Geometry: final body of the model. Coordinates: model frame, mm. A direction names the side the tool comes from. Give positions to 0.01 mm unless a question says otherwise; leave off trailing zeros. Write each loop counter-clockwise with the first axis right and the second up, starting at its lowest first coordinate (ties: lowest second). Pieces come first, ordered by that corner, then holes. Notation, with made-up numbers: (11, 70) - (53, 70) arc R33 cw to (53, 106) - close; hole circle Ø3 at (-21.5, -19.75). An arc over 180 degrees is marked (long way). Return JSON: item names as keys, results as strings.
from build123d import *

# Parameters (mm, degrees)
SKETCH1_W                 = 96.9
SKETCH1_H                 = 214
BOSS_EXTRUDE1_DEPTH       = 3
SKETCH2_W                 = 7
SKETCH2_H                 = 214
CUT_EXTRUDE1_DEPTH        = 1.5
F_0_80_TAPPED_HOLE1_D     = 1.19126
F_0_80_TAPPED_HOLE1_DEPTH = 4.0005
F_0_80_TAPPED_HOLE1_TIP   = 0.357890611


with BuildPart() as part:
    # Sketch1 → Boss-Extrude1 (new body)
    with BuildSketch(Plane(origin=(0, 0, 0), x_dir=(1, 0, 0), z_dir=(0, 1, 0))):
        Rectangle(SKETCH1_W, SKETCH1_H)
    extrude(amount=BOSS_EXTRUDE1_DEPTH)

    # Sketch2 → Cut-Extrude1 (cut)
    with BuildSketch(Plane(origin=(0, 3, 0), x_dir=(1, 0, 0), z_dir=(0, 1, 0))):
        with Locations((44.95, 0)):
            Rectangle(SKETCH2_W, SKETCH2_H)
        with Locations((-44.95, 0)):
            Rectangle(SKETCH2_W, SKETCH2_H)
    extrude(amount=-CUT_EXTRUDE1_DEPTH, mode=Mode.SUBTRACT)

    # #0-80 Tapped Hole1
    with Locations(Plane(origin=(0, 3, 0), x_dir=(1, 0, 0), z_dir=(0, 1, 0))):
        with Locations((45.7, -102), (-45.8, -102), (45.7, -79.333333333), (-45.8, -79.333333333), (45.7, -56.666666667), (-45.8, -56.666666667), (45.7, -34), (-45.8, -34), (45.7, -11.333333333), (-45.8, -11.333333333), (45.7, 11.333333333), (-45.8, 11.333333333), (45.7, 34), (-45.8, 34), (45.7, 56.666666667), (-45.8, 56.666666667), (45.7, 79.333333333), (-45.8, 79.333333333), (45.7, 102), (-45.8, 102)):
            Hole(F_0_80_TAPPED_HOLE1_D / 2, depth=F_0_80_TAPPED_HOLE1_DEPTH)
            with Locations((0, 0, -(F_0_80_TAPPED_HOLE1_DEPTH + F_0_80_TAPPED_HOLE1_TIP / 2))):  # 118° drill point
                Cone(0, F_0_80_TAPPED_HOLE1_D / 2, F_0_80_TAPPED_HOLE1_TIP, mode=Mode.SUBTRACT)


solid = part.part
Q1. Material intervals for probe 1 along X at (y, z) = (0.9, -102); probe 2 along X at (y, z) = (2.65, 72), sorted ascending. Write a range as [from, to].
Answer key:
{"probe 1": "x = [-48.45, -46.4], [-45.2, 45.1], [46.3, 48.45]", "probe 2": "x = [-41.45, 41.45]"}
Q2. Set-up query: faces 1 (the flat face through (-45, 1.5, -1)), 2 (the flat face through (-1, 3, -1)), 3 (the flat face through (45, 1.5, -1)). Return all of +Z, -Z, +X, -X, +Y, -Y with unobstructed straight access to the full face (end or side cutting, diameter ignored); none if empty.
Answer key:
{"face 1": "+Z, -Z, -X, +Y", "face 2": "+Z, -Z, +X, -X, +Y", "face 3": "+Z, -Z, +X, +Y"}
Q3. Pin query (flat end, axial travel): P1, Ø3, axis at x = 9.5, z = 49.5, coming from the -Y side; P2, Ø1.2, axis at y = 2.5, z = -8.5, coming from the +X side; P3, Ø2, axis at x = 43, z = -11, coming from the +Y side. Return the tip coordinate at first contact, or that it passes through.
Answer key:
{"P1": "stops at y = 0", "P2": "stops at x = 41.45", "P3": "stops at y = 1.5"}
Q4. Section query A-A, the plane z = 30. Return the cut outline in (x, y).
Answer key:
{"outline": "(-48.45, 0) - (48.45, 0) - (48.45, 1.5) - (41.45, 1.5) - (41.45, 3) - (-41.45, 3) - (-41.45, 1.5) - (-48.45, 1.5) - close"}
